Geometry: final body of the model. Coordinates: model frame, mm. Round coordinates to 2 decimals unless told otherwise and drop trailing zeros. Loops run counter-clockwise (first coordinate to the right, second up) from the corner with the lowest first, then second, coordinate; pieces in that order, holes last. Notation, with made-up numbers: M 0.25,-31 L 52.25,-31 A15 cw 52.25,-6 Z; hole C 2.5,32.25 d6. An arc over 180 degrees is marked long. Return JSON: item names as keys, results as strings.
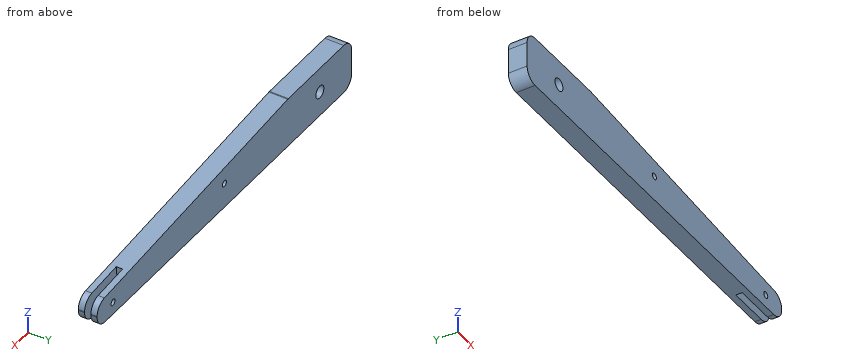
from build123d import *

# Parameters (mm, degrees)
F0_W          = 406.4
F0_H          = 50.8
F0_R          = 3.175
F1_DEPTH      = 19.05
F2_SIZE2      = 25.4
F2_SIZE       = 304.8
F3_R          = 6.35
F4_DEPTH      = 19.051
F5_R          = 3.175
F6_DEPTH      = 19.051
F7_W          = 50.8
F7_H          = 6.35
F8_DEPTH      = 59.062945272
F9_W          = 6.35
F9_H          = 25.4
F10_DEPTH     = 2.54
F11_T1_DEPTH  = 82.55
F11_T3_DEPTH  = 69.85
F11_T5_DEPTH  = 69.85
F11_T7_DEPTH  = 64.7784379794
F11_T9_DEPTH  = 64.7784379794
F11_T11_DEPTH = 21.6912557533


# Not quite as in the source:
# - a fillet or chamfer that OpenCascade refuses, or shapes differently, is made with other operations: its cross-section is extruded or revolved along the edge and cut away or added


with BuildPart() as f1:
    # F0 (on Front) → F1 (new body)
    with BuildSketch(Plane.XZ):
        Rectangle(F0_W, F0_H)
        Circle(F0_R, mode=Mode.SUBTRACT)
    extrude(amount=F1_DEPTH)

    # F2
    f2_edges = [f1.edges().sort_by_distance(p)[0] for p in [
        (203.2, -9.525, 25.4),
    ]]
    f2_side = f1.faces().sort_by_distance((0, -9.525, 25.4))[0]
    chamfer(f2_edges, length=F2_SIZE, length2=F2_SIZE2, reference=f2_side)

    # F3 (on face) → F4 (cut, through all)
    with BuildSketch(Plane.XZ.offset(19.05)):
        with Locations((-152.4, 0)):
            Circle(F3_R)
    extrude(amount=-F4_DEPTH, mode=Mode.SUBTRACT)

    # F5 (on face) → F6 (cut, through all)
    with BuildSketch(Plane.XZ.offset(19.05)):
        with Locations((177.8, -12.7)):
            Circle(F5_R)
    extrude(amount=-F6_DEPTH, mode=Mode.SUBTRACT)

    # F7 (on face) → F8 (cut, through all)
    with BuildSketch(Plane(origin=(1.4013793103, 0, 16.8165517241), x_dir=(0.9965457582, 0, -0.0830454799), z_dir=(0.0830454799, 0, 0.9965457582))):
        with Locations((177.0980980754, -9.525)):
            Rectangle(F7_W, F7_H)
    extrude(amount=-F8_DEPTH, mode=Mode.SUBTRACT)

    # F9 (on face) → F10 (cut)
    with BuildSketch(Plane.YZ.offset(203.2)):
        with Locations((-9.525, -12.7)):
            Rectangle(F9_W, F9_H)
    extrude(amount=-F10_DEPTH, mode=Mode.SUBTRACT)

    # F11: fillet of radius 12.7 on 7 edges, made by hand

    # F11_s2 → F11_t1 (cut)
    with BuildSketch(Plane.XZ.offset(-31.75)):
        with BuildLine():
            ThreePointArc((-190.5, 25.4), (-199.4802561211, 21.6802561211), (-203.2, 12.7))
            Line((-203.2, 12.7), (-203.2, 25.4))
            Line((-203.2, 25.4), (-190.5, 25.4))
        make_face()
        with BuildLine():
            ThreePointArc((-190.5, -25.4), (-199.4802561211, -21.6802561211), (-203.2, -12.7))
            Line((-203.2, -12.7), (-203.2, -25.4))
            Line((-203.2, -25.4), (-190.5, -25.4))
        make_face()
    extrude(amount=F11_T1_DEPTH, mode=Mode.SUBTRACT)

    # F11_s4 → F11_t3 (cut)
    with BuildSketch(Plane.XZ.offset(-19.05)):
        with BuildLine():
            ThreePointArc((190.5, -25.4), (199.4802561211, -21.6802561211), (203.2, -12.7))
            Line((203.2, -12.7), (203.2, -25.4))
            Line((203.2, -25.4), (190.5, -25.4))
        make_face()
    extrude(amount=F11_T3_DEPTH, mode=Mode.SUBTRACT)

    # F11_s6 → F11_t5 (cut)
    with BuildSketch(Plane.XZ.offset(-31.75)):
        with BuildLine():
            ThreePointArc((203.2, -12.7), (199.4802561211, -21.6802561211), (190.5, -25.4))
            Line((190.5, -25.4), (203.2, -25.4))
            Line((203.2, -25.4), (203.2, -12.7))
        make_face()
    extrude(amount=F11_T5_DEPTH, mode=Mode.SUBTRACT)

    # F11_s8 → F11_t7 (cut)
    with BuildSketch(Plane.XZ.offset(-29.2142189897)):
        with BuildLine():
            ThreePointArc((203.2, -11.6856875959), (199.8457050415, -3.0863970858), (191.5546775941, 0.9704435338))
            Line((191.5546775941, 0.9704435338), (203.2, 0))
            Line((203.2, 0), (203.2, -11.6856875959))
        make_face()
    extrude(amount=F11_T7_DEPTH, mode=Mode.SUBTRACT)

    # F11_s10 → F11_t9 (cut)
    with BuildSketch(Plane.XZ.offset(-16.5142189897)):
        with BuildLine():
            ThreePointArc((203.2, -11.6856875959), (199.8457050415, -3.0863970858), (191.5546775941, 0.9704435338))
            Line((191.5546775941, 0.9704435338), (203.2, 0))
            Line((203.2, 0), (203.2, -11.6856875959))
        make_face()
    extrude(amount=F11_T9_DEPTH, mode=Mode.SUBTRACT)

    # F11_s12 → F11_t11 (cut)
    with BuildSketch(Plane.XZ.offset(-1.3206278767)):
        with BuildLine():
            ThreePointArc((-102.1282511507, 25.4), (-101.6004563739, 25.3890280429), (-101.0735735565, 25.3561311297))
            Line((-101.0735735565, 25.3561311297), (-101.6, 25.4))
            Line((-101.6, 25.4), (-102.1282511507, 25.4))
        make_face()
    extrude(amount=F11_T11_DEPTH, mode=Mode.SUBTRACT)


solid = f1.part
Q1. Section query D-D (z = 22). Output: boundary loops of the cut face in (x, y).
Determined:
{"outline": "M -199.15,-19.05 L -60.8,-19.05 L -60.8,0 L -199.15,0 Z"}
Q2. Section query B-B (x = 158.5). Output: boundary loops of the cut face in (y, z) (3 decimals).
Determined:
{"outline": "M -19.05,-25.4 L -12.7,-25.4 L -12.7,3.725 L -19.05,3.725 Z; M -6.35,-25.4 L 0,-25.4 L 0,3.725 L -6.35,3.725 Z"}
Q3. Section query C-C (x = -65). Output: boundary loops of the cut face in (y, z), plus the area to 3 significant figures.
Determined:
{"outline": "M -19.05,-25.4 L 0,-25.4 L 0,22.35 L -19.05,22.35 Z", "area": "910 mm^2"}
Q4. Pin query (flat end, axial travel): pin 1 (5 mm diameter, centred on x = 111.5, y = -10, fed in from +Z); pin 2 (6 mm diameter, centred on y = -4.5, z = 19.5, fed in from -X); pin 3 (2 mm diameter, centred on y = -3, z = -5.5, fed in from +X). Return the tip coordinate at first contact, or that it passes through.
Determined:
{"pin 1": "stops at z = 7.85", "pin 2": "stops at x = -202.62", "pin 3": "stops at x = 202.09"}
Q5. Section query A-A (x = -152.4). Output: boundary loops of the cut face in (y, z), plus the area to 3 significant figures.
Determined:
{"outline": "M -19.05,-25.4 L 0,-25.4 L 0,-6.35 L -19.05,-6.35 Z; M -19.05,6.35 L 0,6.35 L 0,25.4 L -19.05,25.4 Z", "area": "726 mm^2"}
Q6. Material intervals for L1, parallel to Y at x = 157, z = 2.5; L2, parallel to Z at x = -152.4, y = -14; L3, parallel to Z at x = 0, y = -13.75 (3 decimals), sorted ascending.
Determined:
{"L1": "y = -19.05 to -12.7, -6.35 to 0", "L2": "z = -25.4 to -6.35, 6.35 to 25.4", "L3": "z = -25.4 to -3.175, 3.175 to 16.933"}
